Autodesk Inventor part; units mm, degrees
ref_plane "YZ Plane" through (0, 0, 0) normal (1, 0, 0) x (0, 1, 0)
ref_plane "XZ Plane" through (0, 0, 0) normal (0, 1, 0) x (-1, 0, 0)
ref_plane "XY Plane" through (0, 0, 0) normal (0, 0, 1) x (1, 0, 0)
sketch "Sketch1" plane through (0, 0, 0) normal (0, 0, 1) x (1, 0, 0)
  circle A0 centre (0, 0) radius 11.1125
  circle A1 centre (0, 0) radius 15.875
  dimension "d0" = 22.225
  dimension "d1" = 31.75
extrude "Extrusion1" add sketch "Sketch1" along normal blind 7.62
chamfer "Chamfer1" distance 0.7937 angle 45 1 edges at (-15.875, 0, 0)
chamfer "Chamfer2" distance 3.175 angle 45 2 edges at (-11.1125, 0, 7.62) (-11.1125, 0, 0)
equation "\"d1\" = Wheel_OD"
properties part number "Tire" material "Rubber, Silicone"
Source: CAD feature listing. Evaluate the final solid. Frame: model axes, mm. Round coordinates to 2 decimals unless told otherwise and drop trailing zeros. Loops run counter-clockwise (first coordinate to the right, second up) from the corner with the lowest first, then second, coordinate; pieces in that order, holes last.
1. Section query A-A on x = 0. Output: boundary loops of the cut face in (y, z) (1 decimal).
2. Mould query, pull axis Y, two halves, no side actions, for faces 1 (the conical face through (-2.45, -11.04, 4.64)), 2 (the cylindrical face through (-3.441, 15.497, 4.159)), 3 (the flat face through (-11.83, 8.31, 7.62)). Classes: released by +Y, released by -Y, zero draft, split by the parting line, or undercut.
3. Ray query, L1, parallel to Y at x = 0, z = 3.7 (1 decimal); L2, parallel to Y at x = -7.5, z = 6.75; L3, parallel to X at y = 0.5, z = 0.5. Return the intervals inside material, ascending.
4. Contact query for flat-ended pins moving along their axis: pin 1 (3 mm diameter, centred on y = -10, z = 6, fed in from +X); pin 2 (2 mm diameter, centred on y = 10, z = 4.5, fed in from +X); pin 3 (3 mm diameter, centred on x = 11.5, z = 6, fed in from -Y). Output: stop coordinate, or through.
Answers below:
1. outline: (-15.9, 0.8) - (-15.1, 0) - (-14.3, 0) - (-11.1, 3.2) - (-11.1, 4.4) - (-14.3, 7.6) - (-15.9, 7.6) - close; (11.1, 3.2) - (14.3, 0) - (15.1, 0) - (15.9, 0.8) - (15.9, 7.6) - (14.3, 7.6) - (11.1, 4.4) - close
2. face 1: undercut
2. face 2: split by the parting line
2. face 3: zero draft
3. L1: y = -15.9 to -11.1, 11.1 to 15.9
3. L2: y = -13.99 to -11.13, 11.13 to 13.99
3. L3: x = -15.57 to -13.78, 13.78 to 15.57
4. pin 1: stops at x = 13.41
4. pin 2: stops at x = 13.08
4. pin 3: stops at y = -12.33
